```python
from build123d import *

# Parameters (mm, degrees)
SKETCH132_W     = 11.2
SKETCH132_H     = 7.21
PAD065_DEPTH    = 1.8
SKETCH135_W     = 1.7
SKETCH135_H     = 1.7
POCKET058_DEPTH = 1.6
SKETCH136_W     = 5.2
SKETCH136_H     = 5.2
PAD066_DEPTH    = 2


with BuildPart() as part:
    # Sketch132 (on YZ_Plane of Origin) → Pad065 (new body)
    with BuildSketch(Plane.YZ):
        with Locations((17.348932, 9.405)):
            Rectangle(SKETCH132_W, SKETCH132_H)
    extrude(amount=PAD065_DEPTH)

    # Sketch135 (on YZ_Plane of Origin) → Pocket058 (cut)
    with BuildSketch(Plane.YZ.offset(1.8)):
        with Locations((17.348932, 8.775)):
            Rectangle(SKETCH135_W, SKETCH135_H)
    extrude(amount=-POCKET058_DEPTH, mode=Mode.SUBTRACT)

    # Sketch136 (on YZ_Plane of Origin) → Pad066 (join)
    with BuildSketch(Plane.YZ):
        with Locations((17.348932, 9.405)):
            Rectangle(SKETCH136_W, SKETCH136_H)
    extrude(amount=-PAD066_DEPTH)


with BuildPart() as part_1:
    # Body019 placement: moved
    add(part.part.moved(Location((-27.48, 0, 0))))


solid = part_1.part
```
Here's how the part is built. I have some questions about the finished solid (model axes, mm). A direction names the side the tool comes from. Coordinates: 2 decimals unless noted, no trailing zeros. Order: outer loops, then holes, each group sorted by start corner. A loop starts at its lowest first (then second) coordinate and runs counter-clockwise, first axis right, second up.
1) We'd pull the mould along Y, two halves only. Please class faces 4 (the face through (-26, 17, 9.625)), 5 (the face through (-27.48, 17.3, 12.7)), 6 (the face through (-28, 19.949, 9)): +Y half, -Y half, draft (parallel to the pull), parting line (faces both ways), or undercut.
2) Which directions (+Z, -Z, +X, -X, +Y, -Y) give clear straight access to the entire face, cutting with the end or side of a thin tool? Please do faces 1 (the face through (-26, 18.199, 9)), 2 (the face through (-28, 17, 12.005)), 3 (the face through (-28, 14.749, 9)).
3) Imagine slicing it at C-C on z = 10.25. List the corners of the cut face in (x, y) for me, and give its area (3 significant figures).
4) Will these pins go through, and if not, where does the flat tip stop? pin 1 (1.5 mm diameter, centred on x = -28, y = 16.5, fed in from -Z); pin 2 (1.6 mm diameter, centred on x = -28.5, y = 17, fed in from -Z) (3 decimals); pin 3 (1 mm diameter, centred on x = -28.5, z = 8, fed in from +Y); pin 4 (1.6 mm diameter, centred on x = -28.5, z = 9.5, fed in from -Y).
5) Imagine slicing it at B-B on x = -26.5. List the corners of the cut face in (y, z) for me (3 decimals), and give its area (3 significant figures).
6) Imagine slicing it at A-A on y = 16.75. List the corners of the cut face in (x, z) for me (3 decimals).
7) Imagine slicing it at D-D on z = 9. List the corners of the cut face in (x, y) for me.
8) I need wall thicknesses on line 1 (Y direction, x = -26.35, z = 8); line 2 (X direction, y = 14.5, z = 11.75); line 3 (Y direction, x = -29.15, z = 8.5). Which ranges of each line are inside material? Lowest first, please.
Response values:
1. face 4: undercut
1. face 5: draft
1. face 6: +Y half
2. face 1: +X
2. face 2: +Z, -X, +Y, -Y
2. face 3: +Z, -Z, -X, -Y
3. outline: (-29.48, 14.75) - (-27.48, 14.75) - (-27.48, 11.75) - (-25.68, 11.75) - (-25.68, 22.95) - (-27.48, 22.95) - (-27.48, 19.95) - (-29.48, 19.95) - close
3. area: 30.6 mm2
4. pin 1: stops at z = 5.8
4. pin 2: stops at z = 6.805
4. pin 3: stops at y = 19.95
4. pin 4: stops at y = 14.75
5. outline: (11.749, 5.8) - (22.949, 5.8) - (22.949, 13.01) - (11.749, 13.01) - close; hole (16.499, 7.925) - (18.199, 7.925) - (18.199, 9.625) - (16.499, 9.625) - close
5. area: 77.9 mm2
6. outline: (-29.48, 6.805) - (-27.48, 6.805) - (-27.48, 5.8) - (-25.68, 5.8) - (-25.68, 7.925) - (-27.28, 7.925) - (-27.28, 9.625) - (-25.68, 9.625) - (-25.68, 13.01) - (-27.48, 13.01) - (-27.48, 12.005) - (-29.48, 12.005) - close
7. outline: (-29.48, 14.75) - (-27.48, 14.75) - (-27.48, 11.75) - (-25.68, 11.75) - (-25.68, 16.5) - (-27.28, 16.5) - (-27.28, 18.2) - (-25.68, 18.2) - (-25.68, 22.95) - (-27.48, 22.95) - (-27.48, 19.95) - (-29.48, 19.95) - close
8. line 1: y = 11.75 to 16.5, 18.2 to 22.95
8. line 2: x = -27.48 to -25.68
8. line 3: y = 14.75 to 19.95
